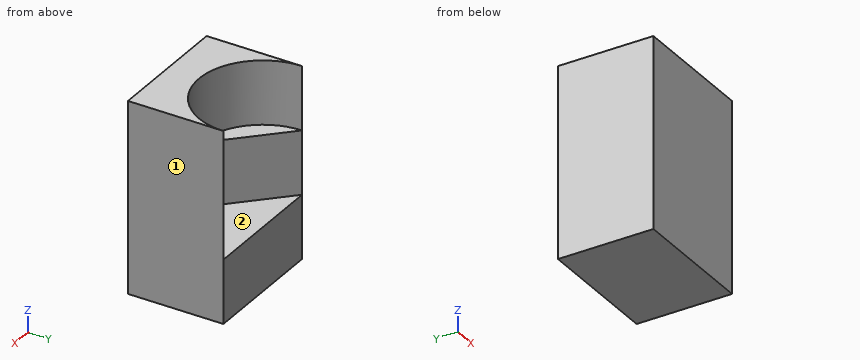
Autodesk Inventor part; units mm, degrees
ref_plane "YZ Plane" through (0, 0, 0) normal (1, 0, 0) x (0, 1, 0)
ref_plane "XZ Plane" through (0, 0, 0) normal (0, 1, 0) x (-1, 0, 0)
ref_plane "XY Plane" through (0, 0, 0) normal (0, 0, 1) x (1, 0, 0)
sketch "草圖1" plane through (0, 0, 0) normal (0, 0, 1) x (1, 0, 0)
  line L0 (0, 0) -> (40, 0)
  line L1 (40, 0) -> (40, 30)
  line L2 (40, 30) -> (0, 30)
  line L3 (0, 30) -> (0, 0)
  dimension "d0" = 40
  dimension "d1" = 30
extrude "擠出1" add sketch "草圖1" along normal blind 20
sketch "草圖2" plane through (0, 0, 20) normal (0, 0, 1) x (1, 0, 0)
  line L0 (0, 30) -> (0, 0)
  line L1 (0, 0) -> (40, 0)
  line L2 (40, 30) -> (40, 0)
  line L3 (40, 0) -> (0, 0)
  line L4 (0, 0) -> (0, 30)
  line L5 (40, 30) -> (0, 30) construction
  line L6 (0, 30) -> (20, 10)
  line L7 (20, 10) -> (40, 30)
  dimension "d4" = 20
  dimension "d5" = 20
extrude "擠出2" add sketch "草圖2" along normal blind 20
sketch "草圖3" plane through (0, 0, 40) normal (0, 0, 1) x (1, 0, 0)
  line L0 (40, 30) -> (20, 10) construction
  arc A0 (0, 29.9839) -> (40, 30) centre (20, 30) ccw
  line L1 (0, 30) -> (0, 0)
  line L2 (0, 29.9839) -> (0, 0)
  line L3 (0, 0) -> (40, 0)
  line L4 (40, 0) -> (40, 30)
  line L5 (40, 0) -> (40, 30)
extrude "擠出3" add sketch "草圖3" along normal blind 20
properties part number "38 (51433.628 mm^3)"
The listing builds one solid part. Answer for the finished solid, in the listing's coordinates (mm). Face numbers are marked on the shaded views. A direction names the side the tool comes from. Give positions to 0.01 mm unless a question says otherwise; leave off trailing zeros. Loops run counter-clockwise (first coordinate to the right, second up) from the corner with the lowest first, then second, coordinate; pieces in that order, holes last. Notation, with made-up numbers: (45.5, 26) - (95.5, 26) arc R23 cw to (95.5, 59) - close; hole circle Ø11 at (51.25, 85.5). An arc over 180 degrees is marked (long way). Answer as a JSON object with one key per item and string values.
1. For the marked faces 1 and 2, determine the directions among +Z, -Z, +X, -X, +Y, -Y from which every point of the face is accessible in a straight line to the end or side of a thin tool.
Determined:
{"face 1": "+Z, -Z, +X, +Y, -Y", "face 2": "+Z, +Y"}
2. A cutting plane is placed at C-C (z = 27.5). Write down the section's boundary in (x, y).
Determined:
{"outline": "(0, 0) - (40, 0) - (40, 30) - (20, 10) - (0, 30) - close"}
3. A cutting plane is placed at B-B (y = 23). Write down the section's boundary in (x, z) (3 decimals), then the cut area to 3 significant figures.
Determined:
{"outline": "(0, 0) - (40, 0) - (40, 60) - (38.735, 60) - (38.735, 40) - (33, 40) - (33, 20) - (7, 20) - (7, 40) - (1.265, 40) - (1.265, 60) - (0, 60) - close", "area": "1,130 mm²"}
4. A cutting plane is placed at A-A (x = 8). Write down the section's boundary in (y, z).
Determined:
{"outline": "(0, 0) - (30, 0) - (30, 20) - (22, 20) - (22, 40) - (14, 40) - (14, 60) - (0, 60) - close"}
5. Find the intervals of material crossed by L1, parallel to Z at x = 36.5, y = 28.5; L2, parallel to X at y = 20, z = 22; L3, parallel to X at y = 17, z = 51, in increasing order. Write a range as [from, to].
Determined:
{"L1": "[0, 20]", "L2": "[0, 10], [30, 40]", "L3": "[0, 4.8], [35.2, 40]"}
6. Flat-ended cylindrical pins translate along their axes: pin 1 Ø16 at (x, y) = (27.5, 21.5) entering from +Z; pin 2 Ø6 at (x, y) = (25, 23) entering from +Z; pin 3 Ø4 at (x, z) = (35, 50.5) entering from +Y; pin 4 Ø6 at (x, z) = (33.5, 8) entering from -Y. Find the tip coordinate at first contact, or state that the pin passes through.
Determined:
{"pin 1": "z = 40", "pin 2": "z = 20", "pin 3": "y = 19.46", "pin 4": "y = 0"}
7. A cutting plane is placed at D-D (y = 16.5). Write down the section's boundary in (x, z), then the cut area to 3 significant figures.
Determined:
{"outline": "(0, 0) - (40, 0) - (40, 60) - (34.76, 60) - (34.76, 40) - (26.5, 40) - (26.5, 20) - (13.5, 20) - (13.5, 40) - (5.24, 40) - (5.24, 60) - (0, 60) - close", "area": "1,550 mm²"}
